```python
from build123d import *

# Parameters (mm, degrees)
SKETCH1_W           = 270
SKETCH1_H           = 260
BOSS_EXTRUDE1_DEPTH = 5
SKETCH2_R           = 3.5
CUT_EXTRUDE1_DEPTH  = 188.483332593
SKETCH3_R           = 15
CUT_EXTRUDE2_DEPTH  = 188.483332593
FILLET1_R           = 5
CUT_EXTRUDE3_DEPTH  = 188.483332593
SKETCH6_W           = 111.9
SKETCH6_H           = 5
BOSS_EXTRUDE2_DEPTH = 5
FILLET2_R           = 10
SKETCH9_W           = 22
SKETCH9_H           = 29
CUT_EXTRUDE5_DEPTH  = 188.483332593
SKETCH10_R          = 1.75
CUT_EXTRUDE6_DEPTH  = 188.483332593
SKETCH11_W          = 100
SKETCH11_H          = 46
CUT_EXTRUDE7_DEPTH  = 188.483332593
SKETCH12_R          = 1.5621
SKETCH12_R_2        = 1.315256363
CUT_EXTRUDE8_DEPTH  = 188.483332593
SKETCH13_W          = 40
SKETCH13_H          = 20
CUT_EXTRUDE9_DEPTH  = 188.483332593
FILLET3_R           = 3
FILLET6_R           = 5
FILLET7_R           = 5


with BuildPart() as part:
    # Sketch1 → Boss-Extrude1 (new body)
    with BuildSketch(Plane.XY):
        Rectangle(SKETCH1_W, SKETCH1_H)
    extrude(amount=BOSS_EXTRUDE1_DEPTH)

    # Sketch2 → Cut-Extrude1 (cut, through all)
    with BuildSketch(Plane(origin=(0, 0, 0), x_dir=(-1, 0, 0), z_dir=(0, 0, -1))):
        with Locations((120, -115)):
            Circle(SKETCH2_R)
        with Locations((86, 90)):
            Circle(SKETCH2_R)
        with Locations((-121, -116)):
            Circle(SKETCH2_R)
    extrude(amount=-CUT_EXTRUDE1_DEPTH, mode=Mode.SUBTRACT)

    # Sketch3 → Cut-Extrude2 (cut, through all)
    with BuildSketch(Plane.XY.offset(5)):
        with Locations((90.172367877, -116)):
            Circle(SKETCH3_R)
    extrude(amount=-CUT_EXTRUDE2_DEPTH, mode=Mode.SUBTRACT)

    # Fillet1
    fillet1_edges = [part.edges().sort_by_distance(p)[0] for p in [
        (135, -130, 2.5),
        (-135, -130, 2.5),
        (-135, 130, 2.5),
        (135, 130, 2.5),
    ]]
    fillet(fillet1_edges, radius=FILLET1_R)

    # Sketch4 → Cut-Extrude3 (cut, through all)
    with BuildSketch(Plane(origin=(0, 0, 0), x_dir=(-1, 0, 0), z_dir=(0, 0, -1))):
        with BuildLine():
            Line((95.6, 100), (135, 100))
            Line((135, 100), (135, 125))
            ThreePointArc((135, 125), (133.535533906, 128.535533906), (130, 130))
            Line((130, 130), (-130, 130))
            ThreePointArc((-130, 130), (-133.535533906, 128.535533906), (-135, 125))
            Line((-135, 125), (-135, 100))
            Line((-135, 100), (90.2, 100))
            Line((90.2, 100), (95.6, 100))
        make_face()
    extrude(amount=-CUT_EXTRUDE3_DEPTH, mode=Mode.SUBTRACT)

    # Sketch6 → Boss-Extrude2 (add)
    with BuildSketch(Plane.XY.offset(5)):
        with Locations((0, 102.5)):
            Rectangle(SKETCH6_W, SKETCH6_H)
    extrude(amount=-BOSS_EXTRUDE2_DEPTH)

    # Fillet2
    fillet2_edges = [part.edges().sort_by_distance(p)[0] for p in [
        (-135, 100, 2.5),
        (135, 100, 2.5),
    ]]
    fillet(fillet2_edges, radius=FILLET2_R)

    # Sketch9 → Cut-Extrude5 (cut, through all)
    with BuildSketch(Plane.XY.offset(5)):
        with Locations((-112.5, 64)):
            Rectangle(SKETCH9_W, SKETCH9_H)
    extrude(amount=-CUT_EXTRUDE5_DEPTH, mode=Mode.SUBTRACT)

    # Sketch10 → Cut-Extrude6 (cut, through all)
    with BuildSketch(Plane(origin=(0, 0, 0), x_dir=(-1, 0, 0), z_dir=(0, 0, -1))):
        with Locations((-46.46, 12.46)):
            Circle(SKETCH10_R)
        with Locations((46.46, 12.46)):
            Circle(SKETCH10_R)
        with Locations((-46.46, -42.46)):
            Circle(SKETCH10_R)
        with Locations((46.46, -42.46)):
            Circle(SKETCH10_R)
    extrude(amount=-CUT_EXTRUDE6_DEPTH, mode=Mode.SUBTRACT)

    # Sketch11 → Cut-Extrude7 (cut, through all)
    with BuildSketch(Plane.XY.offset(5)):
        with Locations((0, -15.253546855)):
            Rectangle(SKETCH11_W, SKETCH11_H)
    extrude(amount=-CUT_EXTRUDE7_DEPTH, mode=Mode.SUBTRACT)

    # Sketch12 → Cut-Extrude8 (cut, through all)
    with BuildSketch(Plane.XY.offset(5)):
        with Locations((112.46, 4.3944)):
            Circle(SKETCH12_R)
        with Locations((64.1238, -3.0986)):
            Circle(SKETCH12_R)
        with Locations((69.002292766, 27.9021)):
            Circle(SKETCH12_R)
        with Locations((97.018492766, 27.9021)):
            Circle(SKETCH12_R_2)
        with Locations((112.46, 79.5276)):
            Circle(SKETCH12_R)
        with Locations((64.1238, 79.5276)):
            Circle(SKETCH12_R)
    extrude(amount=-CUT_EXTRUDE8_DEPTH, mode=Mode.SUBTRACT)

    # Sketch13 → Cut-Extrude9 (cut, through all)
    with BuildSketch(Plane(origin=(0, 0, 0), x_dir=(-1, 0, 0), z_dir=(0, 0, -1))):
        with BuildLine():
            Line((33.41898198, 75), (91.408776107, 75))
            ThreePointArc((91.408776107, 75), (93.158776107, 73.25), (91.408776107, 71.5))
            Line((91.408776107, 71.5), (33.41898198, 71.5))
            ThreePointArc((33.41898198, 71.5), (31.66898198, 73.25), (33.41898198, 75))
        make_face()
        with BuildLine():
            Line((33.41898198, 51.5), (91.408776107, 51.5))
            ThreePointArc((91.408776107, 51.5), (93.158776107, 49.75), (91.408776107, 48))
            Line((91.408776107, 48), (33.41898198, 48))
            ThreePointArc((33.41898198, 48), (31.66898198, 49.75), (33.41898198, 51.5))
        make_face()
        with Locations((-3.530791298, 64)):
            Rectangle(SKETCH13_W, SKETCH13_H)
        with Locations((-3.530791298, -99)):
            Rectangle(SKETCH13_W, SKETCH13_H)
        with BuildLine():
            Line((33.41898198, -86.5), (91.408776107, -86.5))
            ThreePointArc((91.408776107, -86.5), (93.158776107, -84.75), (91.408776107, -83))
            Line((91.408776107, -83), (33.41898198, -83))
            ThreePointArc((33.41898198, -83), (31.66898198, -84.75), (33.41898198, -86.5))
        make_face()
        with BuildLine():
            Line((33.41898198, -110), (91.408776107, -110))
            ThreePointArc((91.408776107, -110), (93.158776107, -108.25), (91.408776107, -106.5))
            Line((91.408776107, -106.5), (33.41898198, -106.5))
            ThreePointArc((33.41898198, -106.5), (31.66898198, -108.25), (33.41898198, -110))
        make_face()
    extrude(amount=-CUT_EXTRUDE9_DEPTH, mode=Mode.SUBTRACT)

    # Fillet3
    fillet3_edges = [part.edges().sort_by_distance(p)[0] for p in [
        (-55.95, 100, 2.5),
        (55.95, 100, 2.5),
    ]]
    fillet(fillet3_edges, radius=FILLET3_R)

    # Fillet6
    fillet6_edges = [part.edges().sort_by_distance(p)[0] for p in [
        (-16.469208702, 74, 2.5),
        (-16.469208702, 54, 2.5),
        (23.530791298, 54, 2.5),
        (23.530791298, 74, 2.5),
    ]]
    fillet(fillet6_edges, radius=FILLET6_R)

    # Fillet7
    fillet7_edges = [part.edges().sort_by_distance(p)[0] for p in [
        (23.530791298, -109, 2.5),
        (23.530791298, -89, 2.5),
        (-16.469208702, -89, 2.5),
        (-16.469208702, -109, 2.5),
    ]]
    fillet(fillet7_edges, radius=FILLET7_R)


solid = part.part
```
Read the model definition and answer for the solid it produces. Units are mm, in the model's axes. Give positions to 0.01 mm unless a question says otherwise; leave off trailing zeros. Loops run counter-clockwise (first coordinate to the right, second up) from the corner with the lowest first, then second, coordinate; pieces in that order, holes last.
Item 1: Find the intervals of material crossed by line 1 along Y through (x, z) = (15, 2.15); line 2 along Y through (x, z) = (-77.5, 0.75); line 3 along Y through (x, z) = (-36.5, 0.2), in increasing order.
Item 2: The part is cut by section B-B (x = 41). Write down the section's boundary in (y, z).
Item 3: The part is cut by section D-D (z = 2). Give the number of separate pieces and of enclosed holes in the cut face, and give its area (3 significant figures).
Item 4: This flat-tipped pin is pushed along its axis until it touches: pin 1 Ø1.6 at (y, z) = (104, 2.5) entering from -X. Where does it stop, or does it pass through?
Item 5: The part is cut by section A-A (x = -86). Write down the section's boundary in (y, z), and give its area (4 significant figures).
Item 6: The part is cut by section C-C (x = 2). Write down the section's boundary in (y, z).
Item 7: The mould has two halves that part along X. Classify faces 1 (the flat face through (-2, 15, 5)), 2 (the cylindrical face through (-132.15, 96.99, 2.54)), 3 (the cylindrical face through (-87.615, 86.895, 2.465)), 4 (the cylindrical face through (90.75, -101.01, 2.54)): released by +X, released by -X, zero draft, split by the parting line, or undercut.
Taken from the geometry:
1. line 1: y = -130 to -109, -89 to -38.25, 7.75 to 54, 74 to 105
1. line 2: y = -130 to -110, -106.5 to -86.5, -83 to 48, 51.5 to 71.5, 75 to 100
1. line 3: y = -130 to -110, -106.5 to -86.5, -83 to -38.25, 7.75 to 48, 51.5 to 71.5, 75 to 105
2. outline: (-130, 0) - (-38.25, 0) - (-38.25, 5) - (-130, 5) - close; (7.75, 0) - (105, 0) - (105, 5) - (7.75, 5) - close
3. separate pieces: 1
3. enclosed holes: 21
3. area: 54,100 mm2
4. pin 1: stops at x = -55.95
5. outline: (-130, 0) - (-110, 0) - (-110, 5) - (-130, 5) - close; (-106.5, 0) - (-86.5, 0) - (-86.5, 5) - (-106.5, 5) - close; (-83, 0) - (48, 0) - (48, 5) - (-83, 5) - close; (51.5, 0) - (71.5, 0) - (71.5, 5) - (51.5, 5) - close; (75, 0) - (86.5, 0) - (86.5, 5) - (75, 5) - close; (93.5, 0) - (100, 0) - (100, 5) - (93.5, 5) - close
5. area: 1,045 mm2
6. outline: (-130, 0) - (-109, 0) - (-109, 5) - (-130, 5) - close; (-89, 0) - (-38.25, 0) - (-38.25, 5) - (-89, 5) - close; (7.75, 0) - (54, 0) - (54, 5) - (7.75, 5) - close; (74, 0) - (105, 0) - (105, 5) - (74, 5) - close
7. face 1: zero draft
7. face 2: released by -X
7. face 3: undercut
7. face 4: undercut
